For this review, take the finished solid that the model builds, in its own axes (mm). Coordinates: 2 decimals unless noted, no trailing zeros. Loops run counter-clockwise (first coordinate to the right, second up) from the corner with the lowest first, then second, coordinate; pieces in that order, holes last. Notation, with made-up numbers: (-13.5, 60) - (1.5, 60) arc R27 cw to (1.5, 84) - close; hole circle Ø8 at (15, 76). An arc over 180 degrees is marked (long way). Answer as a JSON object with one key per item and string values. Group by question number.
Item 1: To check wall thickness, follow line 1 (Z direction, x = -1.25, y = 24.5); line 2 (X direction, y = 32, z = 0.75); line 3 (X direction, y = 19.5, z = -1.5). State the ranges of each line that lie inside material, in increasing order.
Item 2: We need section A-A (y = 30). Give the boundary of the cut face in (x, z), then the cut area to 3 significant figures.
Item 3: Clearance check with flat-ended pins moving along their axes: pin 1 (1.5 mm diameter, centred on y = 16.5, z = -2, fed in from -X); pin 2 (3 mm diameter, centred on x = -1.5, y = 27, fed in from -Z); pin 3 (1 mm diameter, centred on y = 18.5, z = 2, fed in from +X); pin 4 (2 mm diameter, centred on x = -2.5, y = 35.5, fed in from +Z). State where each tip first meets the part, or that it passes through.
from build123d import *

# Parameters (mm, degrees)
SKETCH1_W     = 3.17119
SKETCH1_H     = 50.8
CHAMFER1_SIZE = 0.508
CHAMFER2_SIZE = 0.508


with BuildPart() as part:
    # Sketch1 → Revolve1 (revolve)
    with BuildSketch(Plane.XY):
        with Locations((1.585595, 25.4)):
            Rectangle(SKETCH1_W, SKETCH1_H)
    revolve(axis=Axis((0, 50.8, 0), (0, -1, 0)))

    # Chamfer1
    chamfer1_edges = [part.edges().sort_by_distance(p)[0] for p in [
        (-3.17119, 0, 0),
    ]]
    chamfer(chamfer1_edges, length=CHAMFER1_SIZE)

    # Chamfer2
    chamfer2_edges = [part.edges().sort_by_distance(p)[0] for p in [
        (-3.17119, 50.8, 0),
    ]]
    chamfer(chamfer2_edges, length=CHAMFER2_SIZE)


solid = part.part
Check sheet entries:
{
 "1": {"line 1": "z = -2.91 to 2.91", "line 2": "x = -3.08 to 3.08", "line 3": "x = -2.79 to 2.79"},
 "2": {"outline": "circle Ø6.34 at (0, 0)", "area": "31.6 mm2"},
 "3": {"pin 1": "stops at x = -2.91", "pin 2": "stops at z = -3.17", "pin 3": "stops at x = 2.79", "pin 4": "stops at z = 2.79"}
}
